Check sheet for the modelled part. Datum: model origin and axes. Units: mm. Face numbers are marked on the shaded views. A direction names the side the tool comes from. Round coordinates to 2 decimals unless told otherwise and drop trailing zeros. Write each loop counter-clockwise with the first axis right and the second up, starting at its lowest first coordinate (ties: lowest second). Pieces come first, ordered by that corner, then holes. Notation, with made-up numbers: (-2, 32) -> (29, 32) arc R15 ccw to (29, 57) -> close; hole circle Ø9 at (-5.75, 0). An arc over 180 degrees is marked (long way). One line per item, written item: value. Start each with the question number.
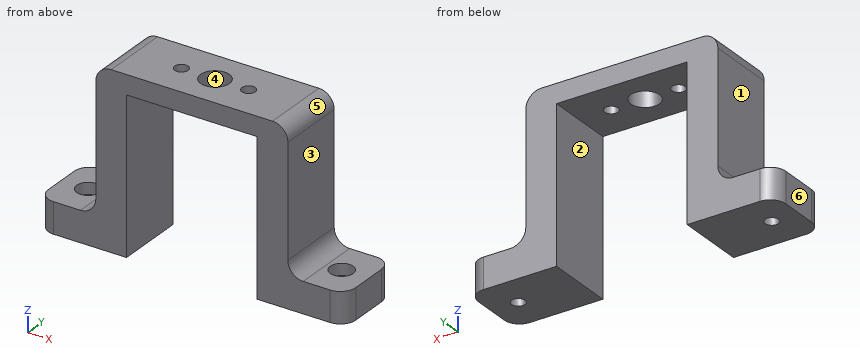
Autodesk Inventor part; units mm, degrees
ref_plane "YZ Plane" through (0, 0, 0) normal (1, 0, 0) x (0, 1, 0)
ref_plane "XZ Plane" through (0, 0, 0) normal (0, 1, 0) x (-1, 0, 0)
ref_plane "XY Plane" through (0, 0, 0) normal (0, 0, 1) x (1, 0, 0)
sketch "Sketch1" plane through (0, 0, 0) normal (0, 0, 1) x (1, 0, 0)
  circle A0 centre (0, 0) radius 3.75
  circle A1 centre (-8.75, 0) radius 1.75
  line L0 (-35, 0) -> (35, 0)
  line L1 (0, 0) -> (0, 3.75)
  circle A2 centre (8.75, 0) radius 1.75
  line L2 (-25, 9) -> (25, 9)
  line L3 (25, 9) -> (25, -9)
  line L4 (25, -9) -> (-25, -9)
  line L5 (-25, -9) -> (-25, 9)
  line L6 (0, -12.6) -> (0, 12.6)
  line L7 (25, 9) -> (17, 9)
  line L8 (17, 9) -> (17, -9)
  line L9 (17, -9) -> (25, -9)
  line L10 (25, -9) -> (25, 9)
  line L11 (-25, 9) -> (-25, -9)
  line L12 (-25, 9) -> (-17, 9)
  line L13 (-17, 9) -> (-17, -9)
  line L14 (-17, -9) -> (-25, -9)
  point P0 (0, 9)
  point P1 (25, 0)
  point P2 (-17, -9)
  point P3 (17, 9)
  point P4 (-17, 9)
  dimension "d2" = 7.5
  dimension "d3" = 3.5
  dimension "d4" = 8.75
  dimension "d5" = 18
  dimension "d6" = 50
  dimension "d9" = 8
extrude "Extrusion1" add sketch "Sketch1" against normal blind 5 contours L0 A2 L8 L4 L6 A0 | A0 L6 L2 L8 L0 A2 | A0 L0 A1 L13 L2 L6 | L6 L4 L13 L0 A1 A0
extrude "Extrusion2" add sketch "Sketch1" against normal blind 45 contours L13 L0 L5 L2 | L2 L3 L0 L8 | L8 L0 L3 L4 | L4 L5 L0 L13
sketch "Sketch2" plane through (25, -9, 0) normal (1, 0, 0) x (0, 0, -1)
  line L0 (5, 0) -> (45, 0)
  line L1 (37, 0) -> (45, 0)
  line L2 (45, 0) -> (45, 18)
  line L3 (45, 18) -> (37, 18)
  line L4 (37, 18) -> (37, 0)
  point P0 (0, 9)
  dimension "d12" = 8
extrude "Extrusion3" add sketch "Sketch2" along normal blind 15
sketch "Sketch3" plane through (25, -9, -37) normal (0, 0, 1) x (1, 0, 0)
  circle A0 centre (8, 9) radius 1.75
  line L0 (-63, 9) -> (28, 9)
  line L1 (0, 0) -> (0, 18)
  point P0 (-25, 9)
  dimension "d15" = 3.5
  dimension "d16" = 8
extrude "Extrusion4" cut sketch "Sketch3" against normal blind 15
mirror "Mirror1" about plane through (0, 0, 0) normal (1, 0, 0) of "Extrusion3", "Extrusion4"
sketch "Sketch4" plane through (0, 0, -45) normal (0, 0, -1) x (-1, 0, 0)
  point P0 (0, 0)
sketch "Sketch5" plane through (25, -9, -37) normal (0, 0, 1) x (1, 0, 0)
  circle A0 centre (8, 9) radius 1.75
  circle A1 centre (8, 9) radius 3
  circle A2 centre (-33.75, 9) radius 1.75
  circle A3 centre (-58, 9) radius 1.75
  circle A4 centre (-58, 9) radius 3
  point P0 (-25, 9)
  dimension "d19" = 6
extrude "Extrusion5" cut sketch "Sketch5" against normal blind 3 contours A1 | A4
fillet "Fillet1" radius 4 8 edges at (25, 0, -37) (25, 0, 0) (-25, 0, 0) (-25, 0, -37) (-40, -9, -41) (-40, 9, -41) (40, -9, -41) (40, 9, -41)
properties part number "Motor _Fixation"
1. Cross-section at B-B (z = -31). Record the cut outline in (x, y), plus the area to 3 significant figures.
2. Cross-section at D-D (x = 33). Record the cut outline in (y, z), plus the area to 4 significant figures.
3. Access from +Z, -Z, +X, -X, +Y, -Y to the whole of each face (thin tool, end or side, straight path). Record for the marked faces 1, 2 and 3.
4. Release check for a two-part mould opening along X. For the marked faces 4, 5 and 6 record: +X half, -X half, draft (parallel to the pull), parting line (faces both ways), or undercut.
5. Cross-section at A-A (x = 0). Record the cut outline in (y, z), plus the area to 3 significant figures.
6. Depth check by flat-ended pin: pin 1 Ø6 at (x, y) = (-15, 1) entering from +Z; pin 2 Ø1.8 at (x, y) = (-34, 1) entering from +Z; pin 3 Ø5.5 at (y, z) = (-4, -18.5) entering from -X; pin 4 Ø4 at (y, z) = (-4, -15) entering from +X. Enter the tip coordinate at first touch or a pass-through.
7. Material ranges on probe 1 along X at (y, z) = (-1.5, -25); probe 2 along X at (y, z) = (0.75, -4.5); probe 3 along Y at (x, z) = (8.75, -1.3), recorded low to high.
8. Cross-section at C-C (y = 0). Give the number of separate pieces and of enclosed holes in the cut face, plus the area to 4 significant figures.
Working result:
1. outline: (-25, -9) -> (-17, -9) -> (-17, 9) -> (-25, 9) -> close; (17, -9) -> (25, -9) -> (25, 9) -> (17, 9) -> close
1. area: 288 mm^2
2. outline: (-9, -45) -> (-1.75, -45) -> (-1.75, -40) -> (-3, -40) -> (-3, -37) -> (-9, -37) -> close; (1.75, -45) -> (9, -45) -> (9, -37) -> (3, -37) -> (3, -40) -> (1.75, -40) -> close
2. area: 108.5 mm^2
3. face 1: +Z, -X, +Y, -Y
3. face 2: -Z, +Y, -Y
3. face 3: +Z, +X, +Y, -Y
4. face 4: undercut
4. face 5: +X half
4. face 6: -X half
5. outline: (-9, -5) -> (-3.75, -5) -> (-3.75, 0) -> (-9, 0) -> close; (3.75, -5) -> (9, -5) -> (9, 0) -> (3.75, 0) -> close
5. area: 52.5 mm^2
6. pin 1: stops at z = 0
6. pin 2: stops at z = -40
6. pin 3: stops at x = -25
6. pin 4: stops at x = 25
7. probe 1: x = -25 to -17, 17 to 25
7. probe 2: x = -25 to -10.33, -7.17 to -3.67, 3.67 to 7.17, 10.33 to 25
7. probe 3: y = -9 to -1.75, 1.75 to 9
8. separate pieces: 6
8. enclosed holes: 0
8. area: 986.5 mm^2
